Design review of the part built by this model. Coordinates are the model's own, in mm. A direction names the side the tool comes from. Round coordinates to 2 decimals unless told otherwise and drop trailing zeros. Loops run counter-clockwise (first coordinate to the right, second up) from the corner with the lowest first, then second, coordinate; pieces in that order, holes last. Notation, with made-up numbers: (83.25, -9.75) - (100.25, -9.75) arc R21 cw to (100.25, 8.25) - close; hole circle Ø2 at (67, 51). An arc over 180 degrees is marked (long way). Return JSON: item names as keys, results as strings. Group by question number.
(1) Wall thickness on L1, parallel to Y at x = -2, z = 6.5: over which ranges is the line inside the solid? List them lowest first. Write a range as [from, to].
(2) We need section A-A, the plane z = -2.5. Write out the cut boundary in (x, y), and give its area (3 significant figures).
(3) We need section C-C, the plane z = 8. Write out the cut boundary in (x, y), and give its area (3 significant figures).
(4) We need section B-B, the plane x = 22. Write out the cut boundary in (y, z), and give its area (3 significant figures).
(5) For faces 1 (the flat face through (-34, 62, 0)), 2 (the cylindrical face through (-27.555, 60.986, -0.846)), list the 3-axis set-ups (+Z, -Z, +X, -X, +Y, -Y) from which the entire face can be reached by the end or side of a thin tool; tool diameter is ignored.
(6) We need section D-D, the plane z = 3. Write out the cut boundary in (x, y), and give its area (3 significant figures).
from build123d import *

# Parameters (mm, degrees)
SKETCH1_W           = 88
SKETCH1_H           = 22
SKETCH1_R           = 6.5
BOSS_EXTRUDE1_DEPTH = 60
SKETCH1_3_R         = 6.5
BOSS_EXTRUDE2_DEPTH = 62


with BuildPart() as part:
    # Sketch1 → Boss-Extrude1 (new body)
    with BuildSketch(Plane(origin=(0, 0, 0), x_dir=(1, 0, 0), z_dir=(0, 1, 0))):
        Rectangle(SKETCH1_W, SKETCH1_H)
        with Locations(Location((-34, 0, 0), (0, 0, 270))):
            Circle(SKETCH1_R, mode=Mode.SUBTRACT)
    extrude(amount=BOSS_EXTRUDE1_DEPTH)

    # Sketch1_3 → Boss-Extrude2 (add)
    with BuildSketch(Plane(origin=(0, 0, 0), x_dir=(1, 0, 0), z_dir=(0, 1, 0))):
        with Locations(Location((-34, 0, 0), (0, 0, 270))):
            Circle(SKETCH1_3_R)
    extrude(amount=BOSS_EXTRUDE2_DEPTH)


solid = part.part
Solutions:
{
 "1": {"L1": "[0, 60]"},
 "2": {"outline": "(-44, 0) - (44, 0) - (44, 60) - (-28, 60) - (-28, 62) - (-40, 62) - (-40, 60) - (-44, 60) - close", "area": "5,300 mm^2"},
 "3": {"outline": "(-44, 0) - (44, 0) - (44, 60) - (-44, 60) - close", "area": "5,280 mm^2"},
 "4": {"outline": "(0, -11) - (60, -11) - (60, 11) - (0, 11) - close", "area": "1,320 mm^2"},
 "5": {"face 1": "+Z, -Z, +X, -X, +Y", "face 2": "+Y"},
 "6": {"outline": "(-44, 0) - (44, 0) - (44, 60) - (-28.23, 60) - (-28.23, 62) - (-39.77, 62) - (-39.77, 60) - (-44, 60) - close", "area": "5,300 mm^2"}
}
